Autodesk Fusion 360 part; units mm, degrees
sketch "Sketch1" plane through (0, 0, 0) normal (0, 0, 1) x (1, 0, 0)
  circle A0 centre (-60, 0) radius 3.75 construction
  circle A1 centre (-60, 0) radius 10 construction
  line L0 (-120, 10) -> (-40.6913, 10)
  line L1 (-120, -10) -> (-40.6913, -10)
  line L2 (-40.6913, 10) -> (-40.6913, -10)
  arc A2 (-120, 10) -> (-120, -10) centre (-120, 0) ccw
  dimension "d1" = 20
  dimension "d2" = 7.5
  dimension "d3" = 60
  dimension "d4" = 20
extrude "Extrude1" add sketch "Sketch1" along normal blind 8 makes body 1
sketch "Sketch2" plane through (0, 0, 0) normal (0, 1, 0) x (1, 0, 0)
  line L0 (-43, -20) -> (-35, -20)
  line L1 (-35, -20) -> (-35, 20)
  line L2 (-35, 20) -> (-43, 20)
  line L3 (-43, 20) -> (-43, -20)
  dimension "d7" = 8
  dimension "d8" = 40
extrude "Extrude2" add sketch "Sketch2" along normal blind 10 and the other way blind 10 separate body makes body 2
copy_body "Body->Comp1" bodies 1 removing the originals makes body 3 in component "section 1 (l4)"
copy_body "Body->Comp2" bodies 2 removing the originals makes body 4 in component "middle bit"
sketch "Sketch3" plane through (0, 0, 8) normal (0, 0, 1) x (-1, 0, 0)
  line L0 (40.6913, -10) -> (120, -10)
  arc A0 (120, -10) -> (120, 10) centre (120, 0) ccw
  line L1 (120, 10) -> (40.6913, 10)
  line L2 (40.6913, 10) -> (40.6913, -10)
  line L3 (25, -10) -> (25, 10)
  line L4 (25, -10) -> (-56.3022, -4.9345)
  line L5 (25, 10) -> (-56.3022, 4.9345)
  line L6 (-58, -11) -> (-72.0708, -11)
  line L7 (-72.0708, -11) -> (-72.0708, -7.0714)
  line L8 (-58, -7.0714) -> (-58, -11)
  arc A1 (-58, -7.1414) -> (-56.3022, -4.9345) centre (-65, 0) ccw
  arc A2 (-56.3022, 4.9345) -> (-72.0708, -7.0714) centre (-65, 0) ccw
  circle A3 centre (-65, 0) radius 6
  dimension "d17" = 20
  dimension "d18" = 90
  dimension "d19" = 12
extrude "Extrude3" add sketch "Sketch3" along normal blind 8 separate body contours L3 L4 L5 L6 L7 L8 A1 A2 makes body 5
sketch "Sketch5" plane through (0, 0, 0) normal (0, 0, 1) x (1, 0, 0)
  circle A0 centre (65.005, -0.1371) radius 6
  line L0 (-25, -10) -> (-25, 10)
  line L1 (-25, 10) -> (56.3881, 4.9373)
  line L2 (-25, -10) -> (56.247, -4.9638)
  line L3 (71.9058, 7.1002) -> (72, 7.1002)
  line L4 (72, 7.1002) -> (72, 11)
  line L5 (72, 11) -> (58.1042, 11)
  line L6 (58.1042, 11) -> (58.1042, 7.1002)
  arc A1 (56.247, -4.9638) -> (71.9058, 7.1002) centre (65.005, -0.1371) ccw
  arc A2 (58.1042, 7.1002) -> (56.3881, 4.9373) centre (65.005, -0.1371) ccw
  dimension "d24" = 20
  dimension "d25" = 12
extrude "Extrude4" add sketch "Sketch5" against normal blind 8 separate body makes body 6
copy_body "Body->Comp3" bodies 5 removing the originals makes body 7 in component "top arm "
copy_body "Body->Comp4" bodies 6 removing the originals makes body 8 in component "bottom arm"
cylinder "CylinderPrimitive1" add diameter 7.7 height 3.5 placed x (1, 0, 0) y (0, 1, 0) z (0, 0, 1) at (-120, 0, 8) bodies 3 in component "section 1 (l4)"
cylinder "CylinderPrimitive2" add diameter 7.7 height 3.5 placed x (0, 1, 0) y (1, 0, 0) z (0, 0, -1) at (-57.218, 0, 0) bodies 3 in component "section 1 (l4)"
sketch "Sketch9" plane through (-0.218, 11, 0) normal (0, 1, 0) x (-1, 0, 0)
  line L0 (-54.2887, 20) -> (-40.218, 20)
  line L1 (-40.218, 20) -> (-40.218, 28)
  line L2 (-40.218, 28) -> (-54.2887, 28)
  line L3 (-54.2887, 28) -> (-54.2887, 20)
  circle A0 centre (-47.1099, 23.7364) radius 2.5
  circle A1 centre (-47.2533, -23.9842) radius 2.5
  dimension "d44" = 5
  dimension "d45" = 5
extrude "Extrude1'" cut sketch "Sketch9" against normal blind 10 contours A0 | A1 sketch seen with x (1, 0, 0) y (0, 1, 0) z (0, 0, 1) at (18, 0, -12) bodies 7 in component "top arm "
combine "Combine1" operation add target body 3 tool bodies 7 8 4 body 7 seen with x (1, 0, 0) y (0, 1, 0) z (0, 0, 1) at (-15.6913, 0, 16) body 8 seen with x (1, 0, 0) y (0, 1, 0) z (0, 0, 1) at (-15.6913, 0, -16) body 4 seen with x (1, 0, 0) y (0, 1, 0) z (0, 0, 1) at (2.3087, 0, 4) in component "section 1 (l4)"
sketch "Sketch10" plane through (0, 0, 7.5) normal (0, 0, 1) x (-1, 0, 0)
  circle A0 centre (122.3087, 0) radius 3.85
  circle A1 centre (122.3087, 0) radius 1.5
  dimension "d50" = 3
extrude "Extrude1''" cut sketch "Sketch10" against normal blind 18 contours A1 sketch seen with x (1, 0, 0) y (0, 1, 0) z (0, 0, 1) at (2.3087, 0, 4) bodies 3 in component "section 1 (l4)"
sketch "Sketch11" plane through (0, 0, -7.5) normal (0, 0, -1) x (1, 0, 0)
  circle A0 centre (-59.5266, 0) radius 3.85
  circle A1 centre (-59.5266, 0) radius 1.5
  dimension "d53" = 3
extrude "Extrude2'" cut sketch "Sketch11" against normal blind 14 contours A1 sketch seen with x (1, 0, 0) y (0, 1, 0) z (0, 0, 1) at (2.3087, 0, 4) bodies 3 in component "section 1 (l4)"
component "section 1 (l4)" placed x (1, 0, 0) y (0, 1, 0) z (0, 0, 1) at (-2.3087, 0, -4)
component "middle bit" placed x (1, 0, 0) y (0, 1, 0) z (0, 0, 1) at (0, 0, 0)
component "top arm " placed x (1, 0, 0) y (0, 1, 0) z (0, 0, 1) at (-18, 0, 12)
component "bottom arm" placed x (1, 0, 0) y (0, 1, 0) z (0, 0, 1) at (-18, 0, -20)
Work out the finished part from the listing and answer in its coordinate system (mm). A direction names the side the tool comes from. Give positions to 0.01 mm unless a question says otherwise; leave off trailing zeros. Order: outer loops, then holes, each group sorted by start corner. A loop starts at its lowest first (then second) coordinate and runs counter-clockwise, first axis right, second up. Notation, with made-up numbers: (75, 9.5) -> (120, 9.5) arc R15 cw to (120, 20.5) -> close; hole circle Ø7 at (2.5, 66.25). An arc over 180 degrees is marked (long way). Answer as CSV lines item,"result". Start each with the question number.
(1) Section C-C, the plane x = 47 is taken. Write down the section's boundary in (y, z), plus the area to 3 significant figures.
(2) Section D-D, the plane x = -10.5 is taken. Write down the section's boundary in (y, z), plus the area to 3 significant figures.
(3) For a pull along X with two mould halves and no side action, classify faces 4 (the cylindrical face through (-63.285, -0.835, -5.774)), 5 (the cylindrical face through (-132.306, -0.22, -0.056)), 6 (the flat face through (10, 1, -20)) as released by +X, released by -X, zero draft, split by the parting line, or undercut.
(4) Section A-A, the plane x = 19.5 is taken. Write down the section's boundary in (y, z), plus the area to 3 significant figures.
(5) Section B-B, the plane z = -22 is taken. Write down the section's boundary in (x, y) (3 decimals), plus the area to 3 significant figures.
(6) Consider line 1 along X through (y, z) = (0, -4.75); line 2 along Z through (x, y) = (12, -5); line 3 along Z through (x, y) = (-101, 1.25). Determine where each line is inside the solid, lowest interval first.
(7) Each of these flat-tipped pins is pushed along its axis until it touches: pin 1 Ø12 at (y, z) = (0.5, -18.5) entering from +X (3 decimals); pin 2 Ø3.5 at (x, y) = (-59.53, 0) entering from -Z; pin 3 Ø10 at (x, y) = (-108.5, 2) entering from +Z; pin 4 Ø12 at (x, y) = (-109.5, -1) entering from -Z. Where does it stop, or does it pass through?
(8) Which of the six approach directions +Z, -Z, +X, -X, +Y, -Y give full straight-line access (tool end or side, diameter ignored) to faces 1 (the flat face through (-122, -2, 7.5)), 2 (the flat face through (-59, 2, -7.5)), 3 (the flat face through (12, 0, 20))?
Entries:
1,outline,"(-10.14, -28) -> (-6.14, -28) -> (-6.14, -20) -> (-10.14, -20) -> close; (-10, 20) -> (-6, 20) -> (-6, 28) -> (-10, 28) -> close; (5.86, -28) -> (11, -28) -> (11, -20) -> (5.86, -20) -> close; (6, 20) -> (11, 20) -> (11, 21.24) -> (6, 21.24) -> close; (6, 26.23) -> (11, 26.23) -> (11, 28) -> (6, 28) -> close"
1,area,"120 mm²"
2,outline,"(-7.99, -28) -> (7.98, -28) -> (7.98, -20) -> (-7.99, -20) -> close; (-7.98, 20) -> (7.98, 20) -> (7.98, 28) -> (-7.98, 28) -> close"
2,area,"255 mm²"
3,face 4,"undercut"
3,face 5,"released by -X"
3,face 6,"zero draft"
4,outline,"(-6.13, -28) -> (6.11, -28) -> (6.11, -20) -> (-6.13, -20) -> close; (-6.11, 20) -> (6.11, 20) -> (6.11, 28) -> (-6.11, 28) -> close"
4,area,"196 mm²"
5,outline,"(-43, -10) -> (38.247, -4.964) arc R10 ccw (long way) to (53.906, 7.1) -> (54, 7.1) -> (54, 11) -> (40.104, 11) -> (40.104, 7.1) arc R10 ccw to (38.388, 4.937) -> (-43, 10) -> close; hole circle Ø12 at (47.005, -0.137)"
5,area,"1,440 mm²"
6,line 1,"-63.38 to -61.03, -58.03 to -55.68, -43 to -35"
6,line 2,"-28 to -20, 20 to 28"
6,line 3,"-4 to 4"
7,pin 1,"x = 57.005"
7,pin 2,"z = -7.5"
7,pin 3,"z = 4"
7,pin 4,"z = -4"
8,face 1,"+Z, -X, +Y, -Y"
8,face 2,"-Z, -X, +Y, -Y"
8,face 3,"+X, +Y, -Y"
